Here's how the part is built. I have some questions about the finished solid (model axes, mm). Face numbers are marked on the shaded views. A direction names the side the tool comes from. Round coordinates to 2 decimals unless told otherwise and drop trailing zeros. Loops run counter-clockwise (first coordinate to the right, second up) from the corner with the lowest first, then second, coordinate; pieces in that order, holes last. Notation, with made-up numbers: (78.25, 25) - (94.25, 25) arc R10 ccw to (94.25, 42) - close; hole circle Ø8 at (48.5, 24.5). An arc over 180 degrees is marked (long way). Answer as a JSON object with one key per item and string values. Group by question number.
1) I want a section at A-A, the plane x = -19.5. Please give me the cut outline in (y, z), then the cut area to 3 significant figures.
2) Will these pins go through, and if not, where does the flat tip stop? P1, Ø1, axis at x = 48.5, y = 12.5, coming from the -Z side; P2, Ø20, axis at x = -60, y = 1, coming from the +Z side; P3, Ø4, axis at x = 66, y = 24.5, coming from the +Z side.
3) I want a section at D-D, the plane x = 46. Please give me the cut outline in (y, z).
4) I want a section at C-C, the plane y = -5. Please give me the cut outline in (x, z).
5) I want a section at B-B, the plane z = 25. Please give me the cut outline in (x, y), then the cut area to 3 significant figures.
6) If we mould it in two halves opening along X, with no side actions, what happens to the marked faces 4, 5, 6 and 7? For each: pulls with the +X half, pulls with the -X half, needs draft (parallel to the pull), parting line crosses it, or undercut.
7) Which directions (+Z, -Z, +X, -X, +Y, -Y) give clear straight access to the entire face, cutting with the end or side of a thin tool? Please do the marked faces 1, 2 and 3.
8) If I drill on line 1 along X through (y, z) = (0.5, 11.5); line 2 along Y through (x, z) = (23.5, 3); line 3 along X through (y, z) = (20.5, 25.5), over which ranges is the centre line in solid material (lowest first)? Write a range as [from, to].
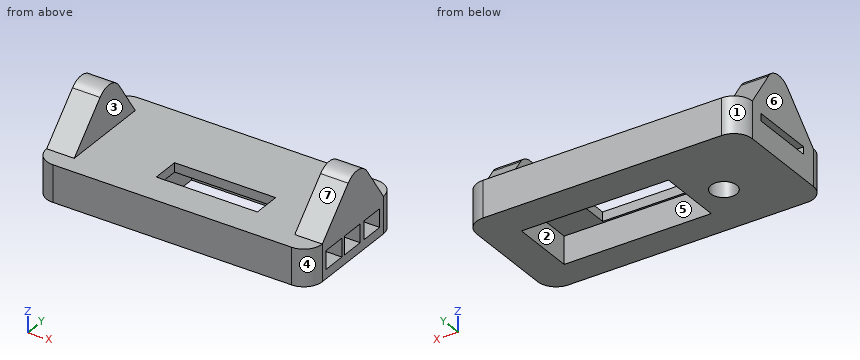
from build123d import *

# Parameters (mm, degrees)
SKETCH1_W           = 150
SKETCH1_H           = 70
BOSS_EXTRUDE1_DEPTH = 20
FILLET1_R           = 10
SKETCH2_W           = 80
SKETCH2_H           = 35
CUT_EXTRUDE1_DEPTH  = 15
SKETCH3_R           = 7
CUT_EXTRUDE2_DEPTH  = 15
SKETCH4_W           = 10
SKETCH4_H           = 13
CUT_EXTRUDE3_DEPTH  = 15
SKETCH6_W           = 4
SKETCH6_H           = 35
CUT_EXTRUDE4_DEPTH  = 25
SKETCH7_W           = 55
SKETCH7_H           = 15
CUT_EXTRUDE5_DEPTH  = 5
BOSS_EXTRUDE3_DEPTH = 15
FILLET2_R           = 10
BOSS_EXTRUDE4_DEPTH = 15


with BuildPart() as part:
    # Sketch1 → Boss-Extrude1 (new body)
    with BuildSketch(Plane.XY):
        with Locations((-0.892857143, 8.973214286)):
            Rectangle(SKETCH1_W, SKETCH1_H)
    extrude(amount=BOSS_EXTRUDE1_DEPTH)

    # Fillet1
    fillet1_edges = [part.edges().sort_by_distance(p)[0] for p in [
        (-75.892857143, 43.973214286, 10),
        (-75.892857143, -26.026785714, 10),
        (74.107142857, -26.026785714, 10),
        (74.107142857, 43.973214286, 10),
    ]]
    fillet(fillet1_edges, radius=FILLET1_R)

    # Sketch2 → Cut-Extrude1 (cut)
    with BuildSketch(Plane(origin=(0, 0, 0), x_dir=(-1, 0, 0), z_dir=(0, 0, -1))):
        with Locations((-15.735916011, 7.430050789)):
            Rectangle(SKETCH2_W, SKETCH2_H)
    extrude(amount=-CUT_EXTRUDE1_DEPTH, mode=Mode.SUBTRACT)

    # Sketch3 → Cut-Extrude2 (cut)
    with BuildSketch(Plane(origin=(0, 0, 0), x_dir=(-1, 0, 0), z_dir=(0, 0, -1))):
        with Locations((40.615191865, 4.17256305)):
            Circle(SKETCH3_R)
    extrude(amount=-CUT_EXTRUDE2_DEPTH, mode=Mode.SUBTRACT)

    # Sketch4 → Cut-Extrude3 (cut)
    with BuildSketch(Plane(origin=(74.107142857, 0, 0), x_dir=(0, 0, -1), z_dir=(1, 0, 0))):
        with Locations((-10, 24.473214286)):
            Rectangle(SKETCH4_W, SKETCH4_H)
        with Locations((-10, 8.473214286)):
            Rectangle(SKETCH4_W, SKETCH4_H)
        with Locations((-10, -6.526785714)):
            Rectangle(SKETCH4_W, SKETCH4_H)
    extrude(amount=-CUT_EXTRUDE3_DEPTH, mode=Mode.SUBTRACT)

    # Sketch6 → Cut-Extrude4 (cut)
    with BuildSketch(Plane.ZY.offset(75.892857143)):
        with Locations((15, 9.473214286)):
            Rectangle(SKETCH6_W, SKETCH6_H)
    extrude(amount=-CUT_EXTRUDE4_DEPTH, mode=Mode.SUBTRACT)

    # Sketch7 → Cut-Extrude5 (cut)
    with BuildSketch(Plane.XY.offset(20)):
        with Locations((6.607142857, -1.526785714)):
            Rectangle(SKETCH7_W, SKETCH7_H)
    extrude(amount=-CUT_EXTRUDE5_DEPTH, mode=Mode.SUBTRACT)

    # Sketch9 → Boss-Extrude3 (add)
    with BuildSketch(Plane.ZY.offset(75.892857143)):
        Polygon((20, 33.973214286), (50.38122201, 13.795245322), (20, -16.026785714), align=None)
    extrude(amount=-BOSS_EXTRUDE3_DEPTH)

    # Fillet2
    fillet2_edges = [part.edges().sort_by_distance(p)[0] for p in [
        (-68.392857143, 13.795245322, 50.38122201),
    ]]
    fillet(fillet2_edges, radius=FILLET2_R)

    # Sketch11 → Boss-Extrude4 (add)
    with BuildSketch(Plane(origin=(74.107142857, 0, 0), x_dir=(0, 0, -1), z_dir=(1, 0, 0))):
        with BuildLine():
            Line((-20, 33.973214286), (-40.105065579, 20.620249447))
            ThreePointArc((-40.105065579, 20.620249447), (-44.527514661, 13.237920805), (-41.577619266, 5.15368001))
            Line((-41.577619266, 5.15368001), (-20, -16.026785714))
            Line((-20, -16.026785714), (-20, 33.973214286))
        make_face()
    extrude(amount=-BOSS_EXTRUDE4_DEPTH)


solid = part.part
Outcome:
{
 "1": {"outline": "(-26.03, 0) - (-10.07, 0) - (-10.07, 15) - (-9.03, 15) - (-9.03, 20) - (-26.03, 20) - close; (5.97, 15) - (24.93, 15) - (24.93, 0) - (43.97, 0) - (43.97, 20) - (5.97, 20) - close", "area": "800 mm^2"},
 "2": {"P1": "z = 15", "P2": "z = 44.48", "P3": "z = 37.27"},
 "3": {"outline": "(-26.03, 0) - (-10.07, 0) - (-10.07, 15) - (24.93, 15) - (24.93, 0) - (43.97, 0) - (43.97, 20) - (-26.03, 20) - close"},
 "4": {"outline": "(-75.89, 0) - (-24.26, 0) - (-24.26, 15) - (-20.89, 15) - (-20.89, 20) - (-60.89, 20) - (-60.89, 31.23) - (-75.89, 31.23) - (-75.89, 17) - (-50.89, 17) - (-50.89, 13) - (-75.89, 13) - close; (34.11, 15) - (55.74, 15) - (55.74, 0) - (74.11, 0) - (74.11, 5) - (59.11, 5) - (59.11, 15) - (74.11, 15) - (74.11, 31.23) - (59.11, 31.23) - (59.11, 20) - (34.11, 20) - close"},
 "5": {"outline": "(-75.89, -11.12) - (-60.89, -11.12) - (-60.89, 30.65) - (-75.89, 30.65) - close; (59.11, -11.12) - (74.11, -11.12) - (74.11, 30.65) - (59.11, 30.65) - close", "area": "1,250 mm^2"},
 "6": {"face 4": "pulls with the +X half", "face 5": "undercut", "face 6": "pulls with the -X half", "face 7": "needs draft"},
 "7": {"face 1": "+Z, -Z, -X, +Y", "face 2": "-Z", "face 3": "+Z, +Y, -Y"},
 "8": {"line 1": "[-75.89, -46.57], [-34.66, -24.26], [55.74, 74.11]", "line 2": "[-26.03, -10.07], [24.93, 43.97]", "line 3": "[-75.89, -60.89], [59.11, 74.11]"}
}
